```python
from build123d import *

# Parameters (mm, degrees)
F1_DEPTH       = 25
F2_SIZE2       = 4
F2_SIZE        = 4
F3_D           = 5.5
F3_CBORE_D     = 9.75
F3_CBORE_DEPTH = 5
F4_D           = 5.5
F4_CBORE_D     = 9.75
F4_CBORE_DEPTH = 5
F5_D           = 5
F6_D           = 5
F9_D           = 3.3
F9_DEPTH       = 7
F9_TIP         = 0.9914200214
F10_D          = 2.3
F10_DEPTH      = 3
F10_TIP        = 0.6909897119


with BuildPart() as f1:
    # F0 (on Top) → F1 (new body)
    with BuildSketch(Plane.XY):
        Polygon((34.59903365, 12.0471221954), (-5.40096635, 12.0471221954), (-5.40096635, -4.9528778046), (-4.40096635, -4.9528778046), (-4.40096635, -10.9528778046), (-5.40096635, -10.9528778046), (-5.40096635, -27.9528778046), (34.59903365, -27.9528778046), align=None)
    extrude(amount=F1_DEPTH)

    # F2
    f2_edges = [f1.edges().sort_by_distance(p)[0] for p in [
        (-5.400966, 12.047122, 12.5),
        (-5.400966, -27.952878, 12.5),
        (34.599034, -27.952878, 12.5),
        (34.599034, 12.047122, 12.5),
    ]]
    chamfer(f2_edges, length=F2_SIZE, length2=F2_SIZE2)

    # F3 (through all)
    with Locations(Plane(origin=(0, 0, 0), x_dir=(1, 0, 0), z_dir=(0, 0, -1))):
        with Locations((6.99903365, 0.1528778046)):
            CounterBoreHole(F3_D / 2, F3_CBORE_D / 2, F3_CBORE_DEPTH)

    # F4 (through all)
    with Locations(Plane(origin=(0, 0, 0), x_dir=(1, 0, 0), z_dir=(0, 0, -1))):
        with Locations((22.59903365, 15.7528778046)):
            CounterBoreHole(F4_D / 2, F4_CBORE_D / 2, F4_CBORE_DEPTH)

    # F5 (through all)
    with Locations(Plane(origin=(0, 0, 0), x_dir=(1, 0, 0), z_dir=(0, 0, -1))):
        with Locations((22.59903365, 0.1528778046)):
            Hole(F5_D / 2)

    # F6 (through all)
    with Locations(Plane(origin=(0, 0, 0), x_dir=(1, 0, 0), z_dir=(0, 0, -1))):
        with Locations((6.99903365, 15.7528778046)):
            Hole(F6_D / 2)

    # F9
    with Locations(Plane(origin=(-5.40096635, 0, 0), x_dir=(0, -1, 0), z_dir=(-1, 0, 0))):
        with Locations((-2.5471221954, 4.8), (18.4528778046, 4.8)):
            Hole(F9_D / 2, depth=F9_DEPTH)
            with Locations((0, 0, -(F9_DEPTH + F9_TIP / 2))):  # 118° drill point
                Cone(0, F9_D / 2, F9_TIP, mode=Mode.SUBTRACT)

    # F10
    with Locations(Plane(origin=(-4.40096635, 0, 0), x_dir=(0, -1, 0), z_dir=(-1, 0, 0))):
        with Locations((7.9528778046, 4.8)):
            Hole(F10_D / 2, depth=F10_DEPTH)
            with Locations((0, 0, -(F10_DEPTH + F10_TIP / 2))):  # 118° drill point
                Cone(0, F10_D / 2, F10_TIP, mode=Mode.SUBTRACT)


solid = f1.part
```
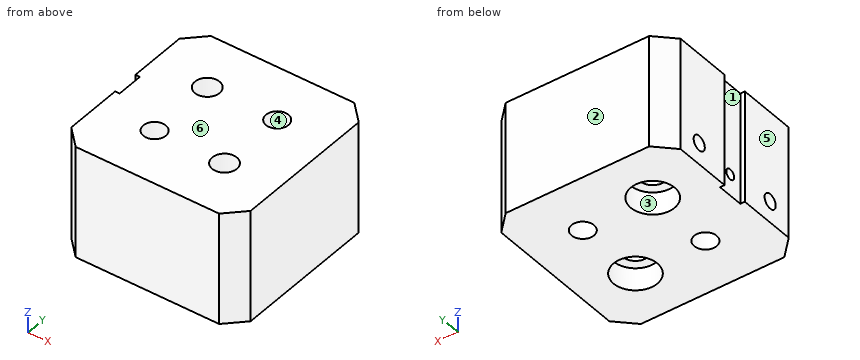
Could you check a few things on this model? Use its own coordinates, in mm. Face numbers are marked on the shaded views. A direction names the side the tool comes from. Round coordinates to 2 decimals unless told otherwise and drop trailing zeros. Loops run counter-clockwise (first coordinate to the right, second up) from the corner with the lowest first, then second, coordinate; pieces in that order, holes last. Notation, with made-up numbers: M -27,-12 L 24,-12 A35 cw 24,22 Z; hole C 49,6 d3. An arc over 180 degrees is marked long. Write item = value, one per line.
1. Which directions (+Z, -Z, +X, -X, +Y, -Y) give clear straight access to the entire face, cutting with the end or side of a thin tool? Please do the marked faces 1, 2 and 3.
Results below:
face_1 = +Z, -Z, -X
face_2 = +Z, -Z, +X, -X, +Y
face_3 = -Z
2. Thinking about a two-plate mould opening in X: for the marked faces 4, 5 and 6, which applies, +X half, -X half, draft (parallel to the pull), parting line (faces both ways), or undercut?
Results below:
face_4 = undercut
face_5 = -X half
face_6 = draft
3. I want a section at B-B, the plane z = 11.5. Write out the boundary of the cut face in (x, y).
Results below:
outline = M -5.4,-23.95 L -1.4,-27.95 L 30.6,-27.95 L 34.6,-23.95 L 34.6,8.05 L 30.6,12.05 L -1.4,12.05 L -5.4,8.05 L -5.4,-4.95 L -4.4,-4.95 L -4.4,-10.95 L -5.4,-10.95 Z; hole C 7,-0.15 d5.5; hole C 7,-15.75 d5; hole C 22.6,-15.75 d5.5; hole C 22.6,-0.15 d5
4. I want a section at A-A, the plane x = 22.5. Write out the boundary of the cut face in (y, z).
Results below:
outline = M -27.95,0 L -20.63,0 L -20.63,5 L -18.5,5 L -18.5,25 L -27.95,25 Z; M -13,5 L -10.88,5 L -10.88,0 L -2.65,0 L -2.65,25 L -13,25 Z; M 2.35,0 L 12.05,0 L 12.05,25 L 2.35,25 Z
5. Will these pins go through, and if not, where does the flat tip stop? P1, Ø5, axis at x = 6, y = 0, coming from the -Z side; P2, Ø6.5, axis at x = 22.6, y = -15.75, coming from the +Z side; P3, Ø1.1, axis at x = -5, z = 7, coming from the +Y side; P4, Ø0.5, axis at x = -5, z = 12.5, coming from the -Y side.
Results below:
P1 = 5
P2 = 25
P3 = 9
P4 = -24.6
6. I want a section at C-C, the plane z = 2.5. Write out the boundary of the cut face in (x, y) (3 decimals).
Results below:
outline = M -5.401,-23.953 L -1.401,-27.953 L 30.599,-27.953 L 34.599,-23.953 L 34.599,8.047 L 30.599,12.047 L -1.401,12.047 L -5.401,8.047 L -5.401,-4.953 L -4.401,-4.953 L -4.401,-10.953 L -5.401,-10.953 Z; hole C 6.999,-0.153 d9.75; hole C 6.999,-15.753 d5; hole C 22.599,-15.753 d9.75; hole C 22.599,-0.153 d5
7. I need wall thicknesses on probe 1 along X at (y, z) = (0, 6.75); probe 2 along Y at (x, z) = (-0.25, 4.8); probe 3 along X at (y, z) = (-18, 3.25). Which ranges of each line are inside material? Lowest first, please.
Results below:
probe_1 = -5.4 to 4.25, 9.74 to 20.1, 25.09 to 34.6
probe_2 = -27.95 to -20.1, -16.8 to 0.9, 4.2 to 12.05
probe_3 = 1.62 to 5.9, 8.09 to 18.27, 26.93 to 34.6
